The listing builds one solid part. Answer for the finished solid, in the listing's coordinates (mm). Face numbers are marked on the shaded views. A direction names the side the tool comes from. Round coordinates to 2 decimals unless told otherwise and drop trailing zeros. Order: outer loops, then holes, each group sorted by start corner. A loop starts at its lowest first (then second) coordinate and runs counter-clockwise, first axis right, second up. Notation, with made-up numbers: (-35.75, 19.5) -> (23.25, 19.5) arc R24 cw to (23.25, 32.5) -> close; hole circle Ø3 at (-25.75, 12.25). An arc over 180 degrees is marked (long way). Return JSON: item names as keys, results as strings. Group by question number.
(1) The part is cut by section A-A (y = -4.5). Determine the outline of the cut face in (x, z), plus the area to 3 significant figures.
(2) The part is cut by section B-B (z = -70). Determine the outline of the cut face in (x, y).
(3) Consider line 1 (Z direction, x = -7.5, y = -9.5); line 2 (Z direction, x = -7.5, y = -7.75); line 3 (Z direction, x = 8.75, y = -9). Determine where each line is inside the solid, lowest interval first. Write a range as [from, to].
(4) The part is cut by section C-C (z = -34). Determine the outline of the cut face in (x, y).
(5) Each of these flat-tipped pins is pushed along its axis until it touches: pin 1 (1.5 mm diameter, centred on x = -3.5, z = 54, fed in from +Y); pin 2 (8 mm diameter, centred on x = 0, z = -14, fed in from +Y); pin 3 (1.8 mm diameter, centred on x = 7.5, z = 97, fed in from -Y); pin 4 (8 mm diameter, centred on y = 1, z = -1, fed in from +X). Where does it stop, or does it pass through?
(6) Which of the six approach directions +Z, -Z, +X, -X, +Y, -Y give full straight-line access (tool end or side, diameter ignored) to the marked faces 1, 2 and 3?
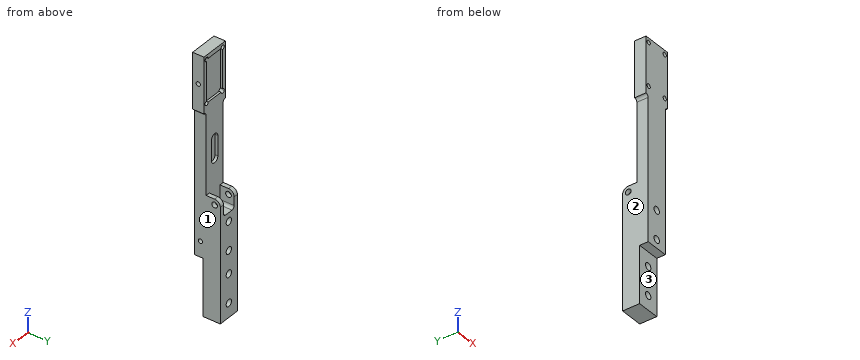
from build123d import *

# Parameters (mm, degrees)
SKETCH1_W               = 140
SKETCH1_H               = 6
BOSS_EXTRUDE1_DEPTH     = 10
SKETCH2_R               = 2
BOSS_EXTRUDE2_DEPTH     = 10
SKETCH6_W               = 2
SKETCH6_H               = 12
CUT_EXTRUDE3_DEPTH      = 98.529482722
CUT_EXTRUDE4_DEPTH      = 10
SKETCH8_W               = 16
SKETCH8_H               = 2
BOSS_EXTRUDE3_DEPTH     = 15
SKETCH9_W               = 20
SKETCH9_H               = 2
BOSS_EXTRUDE4_DEPTH     = 81
CUT_EXTRUDE6_DEPTH      = 102.212647431
CUT_EXTRUDE6_DEPTH_BACK = 102.212647431
SKETCH12_W              = 16
SKETCH12_H              = 12
BOSS_EXTRUDE5_DEPTH     = 40
SKETCH13_R              = 1.5
CUT_EXTRUDE7_DEPTH      = 101.995049384
SKETCH14_W              = 15
SKETCH14_H              = 30
CUT_EXTRUDE8_DEPTH      = 1.5
CUT_EXTRUDE9_DEPTH      = 2
SKETCH16_R              = 2.5
CUT_EXTRUDE10_DEPTH     = 103.097992145
SKETCH17_R              = 2.5
CUT_EXTRUDE11_DEPTH     = 102.212647431
SKETCH18_R              = 1.5
CUT_EXTRUDE12_DEPTH     = 15
SKETCH19_R              = 1.5
CUT_EXTRUDE13_DEPTH     = 15


with BuildPart() as part:
    # Sketch1 → Boss-Extrude1 (new, symmetric)
    with BuildSketch(Plane(origin=(0, 0, 0), x_dir=(0, 0, -1), z_dir=(1, 0, 0))):
        with Locations((-30, -11)):
            Rectangle(SKETCH1_W, SKETCH1_H)
    extrude(amount=BOSS_EXTRUDE1_DEPTH, both=True)

    # Sketch2 → Boss-Extrude2 (add, symmetric)
    with BuildSketch(Plane(origin=(0, 0, 0), x_dir=(0, 0, -1), z_dir=(1, 0, 0))):
        with BuildLine():
            Line((-4, -8), (4, -8))
            Line((4, -8), (40, -8))
            Line((40, -8), (40, 4))
            Line((40, 4), (0, 4))
            ThreePointArc((0, 4), (-2.828427125, 2.828427125), (-4, 0))
            Line((-4, 0), (-4, -8))
        make_face()
        Circle(SKETCH2_R, mode=Mode.SUBTRACT)
    extrude(amount=BOSS_EXTRUDE2_DEPTH, both=True)

    # Sketch6 → Cut-Extrude3 (cut, through all)
    with BuildSketch(Plane.XY.offset(4)):
        with Locations((-9, -2)):
            Rectangle(SKETCH6_W, SKETCH6_H)
        with Locations((9, -2)):
            Rectangle(SKETCH6_W, SKETCH6_H)
    extrude(amount=-CUT_EXTRUDE3_DEPTH, mode=Mode.SUBTRACT)

    # Sketch7 → Cut-Extrude4 (cut)
    with BuildSketch(Plane(origin=(0, 4, 0), x_dir=(1, 0, 0), z_dir=(0, 1, 0))):
        with BuildLine():
            Line((-5, -4), (5, -4))
            Line((5, -4), (5, 6))
            ThreePointArc((5, 6), (4.414213562, 7.414213562), (3, 8))
            Line((3, 8), (-3, 8))
            ThreePointArc((-3, 8), (-4.414213562, 7.414213562), (-5, 6))
            Line((-5, 6), (-5, -4))
        make_face()
    extrude(amount=-CUT_EXTRUDE4_DEPTH, mode=Mode.SUBTRACT)

    # Sketch8 → Boss-Extrude3 (add)
    with BuildSketch(Plane.XY.offset(4)):
        with Locations((0, -7)):
            Rectangle(SKETCH8_W, SKETCH8_H)
    extrude(amount=BOSS_EXTRUDE3_DEPTH)

    # Sketch9 → Boss-Extrude4 (add)
    with BuildSketch(Plane.XY.offset(19)):
        with Locations((0, -7)):
            Rectangle(SKETCH9_W, SKETCH9_H)
    extrude(amount=BOSS_EXTRUDE4_DEPTH)

    # Sketch11 → Cut-Extrude6 (cut, two sides: drawn at the far end of the back side and taken through both)
    with BuildSketch(Plane(origin=(0, -8, 0), x_dir=(1, 0, 0), z_dir=(0, 1, 0)).offset(-CUT_EXTRUDE6_DEPTH_BACK)):
        with BuildLine():
            Line((-10, -59), (-10, -61))
            ThreePointArc((-10, -61), (-8.585786438, -60.414213562), (-8, -59))
            Line((-8, -59), (-8, 40))
            Line((-8, 40), (-10, 40))
            Line((-10, 40), (-10, -59))
        make_face()
        with BuildLine():
            Line((10, 40), (8, 40))
            Line((8, 40), (8, -59))
            ThreePointArc((8, -59), (8.585786438, -60.414213562), (10, -61))
            Line((10, -61), (10, -59))
            Line((10, -59), (10, 40))
        make_face()
    extrude(amount=CUT_EXTRUDE6_DEPTH + CUT_EXTRUDE6_DEPTH_BACK, mode=Mode.SUBTRACT)

    # Sketch12 → Boss-Extrude5 (add)
    with BuildSketch(Plane(origin=(0, 0, -40), x_dir=(-1, 0, 0), z_dir=(0, 0, -1))):
        with Locations((0, -2)):
            Rectangle(SKETCH12_W, SKETCH12_H)
    extrude(amount=BOSS_EXTRUDE5_DEPTH)

    # Sketch13 → Cut-Extrude7 (cut, through all)
    with BuildSketch(Plane(origin=(0, -6, 0), x_dir=(1, 0, 0), z_dir=(0, 1, 0))):
        with Locations(Location((7.5, -97, 0), (0, 0, 270))):
            Circle(SKETCH13_R)
        with Locations(Location((7.5, -67, 0), (0, 0, 270))):
            Circle(SKETCH13_R)
        with Locations(Location((-7.5, -67, 0), (0, 0, 270))):
            Circle(SKETCH13_R)
        with Locations(Location((-7.5, -97, 0), (0, 0, 270))):
            Circle(SKETCH13_R)
    extrude(amount=-CUT_EXTRUDE7_DEPTH, mode=Mode.SUBTRACT)

    # Sketch14 → Cut-Extrude8 (cut)
    with BuildSketch(Plane(origin=(0, -6, 0), x_dir=(1, 0, 0), z_dir=(0, 1, 0))):
        with Locations((0, -82)):
            Rectangle(SKETCH14_W, SKETCH14_H)
    extrude(amount=-CUT_EXTRUDE8_DEPTH, mode=Mode.SUBTRACT)

    # Sketch15 → Cut-Extrude9 (cut)
    with BuildSketch(Plane(origin=(0, -6, 0), x_dir=(1, 0, 0), z_dir=(0, 1, 0))):
        with BuildLine():
            Line((3, -25), (3, -39))
            ThreePointArc((3, -39), (0, -42), (-3, -39))
            Line((-3, -39), (-3, -25))
            ThreePointArc((-3, -25), (0, -22), (3, -25))
        make_face()
    extrude(amount=-CUT_EXTRUDE9_DEPTH, mode=Mode.SUBTRACT)

    # Sketch16 → Cut-Extrude10 (cut, through all)
    with BuildSketch(Plane.XZ.offset(14)):
        with Locations(Location((0, -34, 0), (0, 0, 270))):
            Circle(SKETCH16_R)
        with Locations(Location((0, -14, 0), (0, 0, 270))):
            Circle(SKETCH16_R)
    extrude(amount=-CUT_EXTRUDE10_DEPTH, mode=Mode.SUBTRACT)

    # Sketch17 → Cut-Extrude11 (cut, through all)
    with BuildSketch(Plane.XZ.offset(8)):
        with Locations((0, -70)):
            Circle(SKETCH17_R)
        with Locations((0, -50)):
            Circle(SKETCH17_R)
    extrude(amount=-CUT_EXTRUDE11_DEPTH, mode=Mode.SUBTRACT)

    # Sketch18 → Cut-Extrude12 (cut)
    with BuildSketch(Plane(origin=(8, 0, 0), x_dir=(0, 0, -1), z_dir=(1, 0, 0))):
        with Locations((29.1, -10)):
            Circle(SKETCH18_R)
    extrude(amount=-CUT_EXTRUDE12_DEPTH, mode=Mode.SUBTRACT)

    # Sketch19 → Cut-Extrude13 (cut)
    with BuildSketch(Plane(origin=(10, 0, 0), x_dir=(0, 0, -1), z_dir=(1, 0, 0))):
        with Locations((-79.9, -10)):
            Circle(SKETCH19_R)
    extrude(amount=-CUT_EXTRUDE13_DEPTH, mode=Mode.SUBTRACT)


solid = part.part
Answer below:
{
 "1": {"outline": "(-8, -80) -> (8, -80) -> (8, 4) -> (5, 4) -> (5, -6) arc R2 cw to (3, -8) -> (-3, -8) arc R2 cw to (-5, -6) -> (-5, 4) -> (-8, 4) -> close; hole circle Ø5 at (0, -70); hole circle Ø5 at (0, -50); hole circle Ø5 at (0, -34); hole circle Ø5 at (0, -14)", "area": "1,150 mm²"},
 "2": {"outline": "(-8, -8) -> (-2.5, -8) -> (-2.5, 4) -> (-8, 4) -> close; (2.5, -8) -> (8, -8) -> (8, 4) -> (2.5, 4) -> close"},
 "3": {"line 1": "z = [-40, 65.5], [68.5, 95.5], [98.5, 100]", "line 2": "z = [-80, 65.5], [68.5, 95.5], [98.5, 100]", "line 3": "z = [60.56, 66.17], [67.83, 78.78], [81.02, 96.17], [97.83, 100]"},
 "4": {"outline": "(-8, -14) -> (-2.5, -14) -> (-2.5, 4) -> (-8, 4) -> close; (2.5, -14) -> (8, -14) -> (8, 4) -> (2.5, 4) -> close"},
 "5": {"pin 1": "stops at y = -6", "pin 2": "stops at y = 4", "pin 3": "passes through", "pin 4": "stops at x = 8"},
 "6": {"face 1": "-Z, +X, +Y, -Y", "face 2": "-Z, -X, +Y, -Y", "face 3": "-Z, +X, -X, -Y"}
}
